Part model, mm, in its own coordinate system. Face numbers are marked on the shaded views. A direction names the side the tool comes from. Coordinates: 2 decimals unless noted, no trailing zeros. Order: outer loops, then holes, each group sorted by start corner. A loop starts at its lowest first (then second) coordinate and runs counter-clockwise, first axis right, second up. Notation, with made-up numbers: (58.25, 51.5) - (85.25, 51.5) arc R9 cw to (85.25, 62.5) - close; hole circle Ø5 at (-9.75, 66). An arc over 180 degrees is marked (long way). Use a Markdown table: item, result. Add a question column.
1) Saw through at A-A on x = 0.75. List the corners of the cut face in (y, z) (3 decimals).
2) Wall check: L1, parallel to X at y = 0.15, z = -16.5; L2, parallel to X at y = 1, z = -9; L3, parallel to Y at x = -3, z = -8. Give the ranges that are in metal, low to high. Write a range as [from, to].
3) Saw through at D-D on z = 9.5. List the corners of the cut face in (x, y).
4) Saw through at C-C on z = -7.5. List the corners of the cut face in (x, y), then the cut area to 3 significant figures.
5) Saw through at B-B on y = 0. List the corners of the cut face in (x, z) (3 decimals).
6) Drop a flat-ended pin along its axis: P1, Ø6, axis at x = -3.5, z = -11.5, coming from the -Y side. Give the stop position or say it passes through.
7) Tool access for the marked faces 1 and 2: list every direction of +Z, -Z, +X, -X, +Y, -Y with a clear straight run to the whole face (end or side of a thin tool).
8) Two-plate mould, pull along X, no slides. Class the marked faces 3, 4, 5 and 6: +X half, -X half, draft (parallel to the pull), parting line (faces both ways), or undercut.
Autodesk Inventor part; units mm, degrees
ref_plane "YZ Plane" through (0, 0, 0) normal (1, 0, 0) x (0, 1, 0)
ref_plane "XZ Plane" through (0, 0, 0) normal (0, 1, 0) x (-1, 0, 0)
ref_plane "XY Plane" through (0, 0, 0) normal (0, 0, 1) x (1, 0, 0)
sketch "Sketch1" plane through (0, 0, 0) normal (0, 0, 1) x (1, 0, 0)
  line L0 (-3, 0) -> (3, 0) construction
  line L1 (-3, -2) -> (3, -2)
  line L2 (3, 2) -> (-3, 2)
  arc A0 (-3, 2) -> (-3, -2) centre (-3, 0) ccw
  arc A1 (3, -2) -> (3, 2) centre (3, 0) ccw
  point P0 (0, 0)
  dimension "d0" = 4
  dimension "d1" = 6
extrude "Extrusion1" add sketch "Sketch1" along normal blind 22.225
sketch "Sketch2" plane through (0, 0, 0) normal (0, 0, -1) x (-1, 0, 0)
  circle A0 centre (0, 0) radius 1.25
  circle A1 centre (-3, 0) radius 1.25
  arc A2 (-3, 2) -> (-3, -2) centre (-3, 0) ccw
  circle A3 centre (3, 0) radius 1.25
  dimension "d4" = 2.5
  dimension "d5" = 2.5
  dimension "d8" = 360
extrude "Extrusion2" add sketch "Sketch2" along normal blind 22.225
properties part number "SLEEVE" material "Rubber, Silicone"
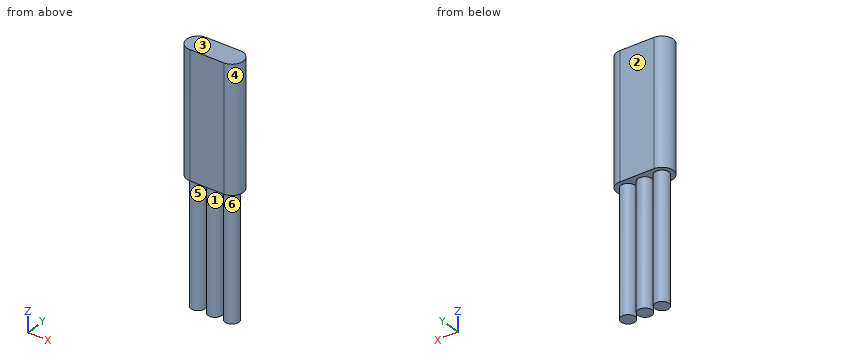
Results are:
| question | item | result |
|---|---|---|
| 1 | outline | (-2, 0) - (-1, 0) - (-1, -22.225) - (1, -22.225) - (1, 0) - (2, 0) - (2, 22.225) - (-2, 22.225) - close |
| 2 | L1 | [-4.24, -1.76], [-1.24, 1.24], [1.76, 4.24] |
| 2 | L2 | [-3.75, -2.25], [-0.75, 0.75], [2.25, 3.75] |
| 2 | L3 | [-1.25, 1.25] |
| 3 | outline | (-3, -2) - (3, -2) arc R2 ccw to (3, 2) - (-3, 2) arc R2 ccw to start |
| 4 | outline | circle Ø2.5 at (-3, 0); circle Ø2.5 at (0, 0); circle Ø2.5 at (3, 0) |
| 4 | area | 14.7 mm2 |
| 5 | outline | (-5, 0) - (-4.25, 0) - (-4.25, -22.225) - (-1.75, -22.225) - (-1.75, 0) - (-1.25, 0) - (-1.25, -22.225) - (1.25, -22.225) - (1.25, 0) - (1.75, 0) - (1.75, -22.225) - (4.25, -22.225) - (4.25, 0) - (5, 0) - (5, 22.225) - (-5, 22.225) - close |
| 6 | P1 | y = -1.25 |
| 7 | face 1 | -Z |
| 7 | face 2 | +Z, -Z, +X, -X, +Y |
| 8 | face 3 | draft |
| 8 | face 4 | +X half |
| 8 | face 5 | undercut |
| 8 | face 6 | undercut |
